Autodesk Inventor part; units mm, degrees
ref_plane "YZ Plane" through (0, 0, 0) normal (1, 0, 0) x (0, 1, 0)
ref_plane "XZ Plane" through (0, 0, 0) normal (0, 1, 0) x (-1, 0, 0)
ref_plane "XY Plane" through (0, 0, 0) normal (0, 0, 1) x (1, 0, 0)
sketch "スケッチ1" plane through (0, 0, 0) normal (0, 0, 1) x (1, 0, 0)
  line L0 (0, 0) -> (6, 0)
  line L1 (6, 0) -> (6, -39)
  line L2 (6, -39) -> (0, -39)
  line L3 (0, -39) -> (0, 0)
  line L4 (6, 0) -> (9, 0)
  circle A0 centre (13.5, -4.5) radius 1.25
  circle A1 centre (-7.5, -4.5) radius 1.25
  circle A2 centre (-7.5, -34.5) radius 1.25
  circle A3 centre (13.5, -34.5) radius 1.25
  circle A4 centre (-7.5, -4.5) radius 3.5
  circle A5 centre (13.5, -4.5) radius 3.5
  circle A6 centre (13.5, -34.5) radius 3.5
  circle A7 centre (-7.5, -34.5) radius 3.5
  line L5 (0, 0) -> (-3, 0)
  line L6 (-3, 0) -> (-8.2059, -1.0719)
  line L7 (-8.2059, -7.9281) -> (-3, -9)
  line L8 (-3, -9) -> (0, -9)
  line L9 (6, -9) -> (9, -9)
  line L10 (9, -9) -> (14.2059, -7.9281)
  line L11 (14.2059, -31.0719) -> (9, -30)
  line L12 (9, -30) -> (6, -30)
  line L13 (0, -30) -> (-3, -30)
  line L14 (-3, -30) -> (-8.2059, -31.0719)
  line L15 (-8.2059, -37.9281) -> (-3, -39)
  line L16 (-3, -39) -> (0, -39)
  line L17 (6, -39) -> (9, -39)
  line L18 (9, -39) -> (14.2059, -37.9281)
  line L19 (-7.5, -34.5) -> (13.5, -34.5) construction
  line L20 (9, 0) -> (14.2059, -1.0719)
  circle A8 centre (0, -10.05) radius 1.05
  circle A9 centre (6, -10.05) radius 1.05
  circle A10 centre (0, -28.95) radius 1.05
  circle A11 centre (6, -28.95) radius 1.05
  point P0 (0, -9)
  point P1 (0, -11.1)
  point P2 (0, -27.9)
  point P3 (6, -27.9)
  point P4 (6, -11.1)
  dimension "d0" = 6
  dimension "d1" = 39
  dimension "d2" = 3
  dimension "d3" = 2.5
  dimension "d4" = 2.5
  dimension "d5" = 2.5
  dimension "d6" = 2.5
  dimension "d7" = 7
  dimension "d8" = 7
  dimension "d9" = 7
  dimension "d10" = 7
  dimension "d11" = 3
  dimension "d12" = 3
  dimension "d13" = 3
  dimension "d14" = 3
  dimension "d15" = 3
  dimension "d16" = 3
  dimension "d19" = 4.5
  dimension "d20" = 4.5
  dimension "d21" = 7.5
  dimension "d22" = 7.5
  dimension "d23" = 3
  dimension "d24" = 7.5
  dimension "d25" = 4.5
  dimension "d26" = 7.5
  dimension "d27" = 4.5
  dimension "d28" = 2.1
  dimension "d29" = 2.1
  dimension "d30" = 2.1
  dimension "d31" = 2.1
extrude "押し出し1" add sketch "スケッチ1" along normal blind 3 contours L0 L1 A9 A11 L2 L3 A10 A8 | L3 L8 L7 A4 L6 L5 | L4 L20 A5 L10 L9 L1 | A4 | A5 | L3 L16 L15 A7 L14 L13 | L12 L11 A6 L18 L17 L1 | A7 | A6
properties part number "シールド根本留め具"
Work out the finished part from the listing and answer in its coordinate system (mm). A direction names the side the tool comes from. Round coordinates to 2 decimals unless told otherwise and drop trailing zeros. Loops run counter-clockwise (first coordinate to the right, second up) from the corner with the lowest first, then second, coordinate; pieces in that order, holes last.
(1) For faces 1 (the flat face through (11.57, -8.47, 1.48)), 2 (the flat face through (3, 0, 1)), 3 (the flat face through (-5.639, -8.457, 1.479)), determine the directions among +Z, -Z, +X, -X, +Y, -Y from which every point of the face is accessible in a straight line to the end or side of a thin tool.
Computed values:
face 1: +Z, -Z, +X
face 2: +Z, -Z, +X, -X, +Y
face 3: +Z, -Z, -X
(2) The part is cut by section A-A, the plane x = 6.5. Give the vertices of the cut face in (y, z).
Computed values:
outline: (-39, 0) - (-30, 0) - (-30, 3) - (-39, 3) - close; (-9, 0) - (0, 0) - (0, 3) - (-9, 3) - close
(3) Find the intervals of material crossed by L1, parallel to Y at x = 9, z = 1.3; L2, parallel to Y at x = 13.5, z = 2.25; L3, parallel to Y at x = 0.75, z = 0.25, in increasing order.
Computed values:
L1: y = -39 to -30, -9 to 0
L2: y = -38.07 to -35.75, -33.25 to -30.93, -8.07 to -5.75, -3.25 to -0.93
L3: y = -39 to -29.68, -28.22 to -10.78, -9.32 to 0
(4) Each of these flat-tipped pins is pushed along its axis until it touches: P1, Ø1.5, axis at y = -20.5, z = 1, coming from the -X side; P2, Ø2, axis at x = -7.5, y = -34.5, coming from the +Z side; P3, Ø1, axis at y = -27.5, z = 2, coming from the +X side. Where does it stop, or does it pass through?
Computed values:
P1: stops at x = 0
P2: passes through
P3: stops at x = 6
(5) The part is cut by section C-C, the plane x = -7.5. Give the vertices of the cut face in (y, z).
Computed values:
outline: (-38.07, 0) - (-35.75, 0) - (-35.75, 3) - (-38.07, 3) - close; (-33.25, 0) - (-30.93, 0) - (-30.93, 3) - (-33.25, 3) - close; (-8.07, 0) - (-5.75, 0) - (-5.75, 3) - (-8.07, 3) - close; (-3.25, 0) - (-0.93, 0) - (-0.93, 3) - (-3.25, 3) - close
(6) The part is cut by section B-B, the plane y = -34.5. Give the vertices of the cut face in (x, z).
Computed values:
outline: (-11, 0) - (-8.75, 0) - (-8.75, 3) - (-11, 3) - close; (-6.25, 0) - (12.25, 0) - (12.25, 3) - (-6.25, 3) - close; (14.75, 0) - (17, 0) - (17, 3) - (14.75, 3) - close
(7) The part is cut by section D-D, the plane z = 1.9. Give the vertices of the cut face in (x, y).
Computed values:
outline: (-8.21, -37.93) - (-3, -39) - (9, -39) - (14.21, -37.93) arc R3.5 ccw to (14.21, -31.07) - (9, -30) - (6, -30) arc R1.05 cw to (6, -27.9) - (6, -11.1) arc R1.05 cw to (6, -9) - (9, -9) - (14.21, -7.93) arc R3.5 ccw to (14.21, -1.07) - (9, 0) - (-3, 0) - (-8.21, -1.07) arc R3.5 ccw to (-8.21, -7.93) - (-3, -9) - (0, -9) arc R1.05 cw to (0, -11.1) - (0, -27.9) arc R1.05 cw to (0, -30) - (-3, -30) - (-8.21, -31.07) arc R3.5 ccw to start; hole circle Ø2.5 at (-7.5, -34.5); hole circle Ø2.5 at (-7.5, -4.5); hole circle Ø2.5 at (13.5, -34.5); hole circle Ø2.5 at (13.5, -4.5)
